Build history of the part. All positions in model axes, mm. A direction names the side the tool comes from. Coordinates: 2 decimals unless noted, no trailing zeros. Loops run counter-clockwise (first coordinate to the right, second up) from the corner with the lowest first, then second, coordinate; pieces in that order, holes last.
(1) Two-plate mould, pull along Y, no slides. Class faces 1 (the face through (41.68, -1.88, -5.96)), 2 (the face through (71.4, -0.1, -13.4)), 3 (the face through (70.4, 6, 5)): pulls with the +Y half, pulls with the -Y half, needs draft (parallel to the pull), parting line crosses it, or undercut.
(2) Slice it at B-B (x = 42). Give the cut face in (y, z), and give its area (3 significant figures).
(3) Slice it at A-A (x = 63). Give the cut face in (y, z), and give its area (3 significant figures).
(4) Wall check: L1, parallel to Y at x = 40.5, z = 3.5; L2, parallel to Z at x = 40, y = -2; L3, parallel to Y at x = 7, z = 0. Give the ranges that are in metal, low to high.
(5) Tool access for faces 4 (the face through (72.16, 6.51, -6.43)), 5 (the face through (35.813, -1.505, 6.777)): list every direction of +Z, -Z, +X, -X, +Y, -Y with a clear straight run to the whole face (end or side of a thin tool).
(6) Flat gauge pins, fed straight in: P1, Ø6, axis at y = 2, z = -0.5, coming from the +X side; P2, Ø6, axis at x = 51, z = 4, coming from the -Y side; P3, Ø4, axis at y = -2.5, z = -2.5, coming from the +X side. Where does each tip first touch, or does it go through?
from build123d import *

# Parameters (mm, degrees)
BOSS_EXTRUDE3_DEPTH = 1.9
FILLET4_R           = 8.6
FILLET5_R           = 0.25
FILLET6_R           = 0.5
FILLET7_R           = 1


with BuildPart() as part:
    # Sketch6 → Boss-Extrude3 (new body)
    with BuildSketch(Plane(origin=(72.3, 0, 0), x_dir=(0, 0, -1), z_dir=(1, 0, 0))):
        with BuildLine():
            Line((-9.834595004, -5.292759782), (0, -9.279892888))
            Line((0, -9.279892888), (9.834595004, -5.292759782))
            ThreePointArc((9.834595004, -5.292759782), (13.4, 0), (9.834595004, 5.292759782))
            Line((9.834595004, 5.292759782), (0, 9.279892888))
            Line((0, 9.279892888), (-9.834595004, 5.292759782))
            ThreePointArc((-9.834595004, 5.292759782), (-13.4, 0), (-9.834595004, -5.292759782))
        make_face()
    extrude(amount=-BOSS_EXTRUDE3_DEPTH)

    # Sketch11 → Revolve1 (revolve)
    with BuildSketch(Plane(origin=(0, 0, 0), x_dir=(-1, 0, 0), z_dir=(0, 0, -1))):
        Polygon((-70.4, 7.131416054), (-70.4, 0), (0, 0), (0, 2), (-8.5, 2.2), (-9.5, 6.85), (-61.4, 7.031165912), (-61.4, 7.1), align=None)
    revolve(axis=Axis((70.4, 0, 0), (-1, 0, 0)))

    # Sketch12 → Hole1 (revolve, cut)
    with BuildSketch(Plane(origin=(72.3, 0, 0), x_dir=(0, 0, -1), z_dir=(0, 1, 0))):
        Polygon((0, 0), (0, 72.3), (1, 72.3), (1, 63.239774349), (6.25, 62.110742091), (6.25, 0), align=None)
    revolve(axis=Axis((78.430023899, 0, 0), (-1, 0, 0)), mode=Mode.SUBTRACT)

    # Fillet4
    fillet4_edges = [part.edges().sort_by_distance(p)[0] for p in [
        (71.35, 9.279892888, 0),
        (71.35, -9.279892888, 0),
    ]]
    fillet(fillet4_edges, radius=FILLET4_R)

    # Fillet5
    fillet5_edges = [part.edges().sort_by_distance(p)[0] for p in [
        (9.060225651, 0, 1),
    ]]
    fillet(fillet5_edges, radius=FILLET5_R)

    # Fillet6
    fillet6_edges = [part.edges().sort_by_distance(p)[0] for p in [
        (70.4, 0, -13.4),
        (70.4, 6.631339679, -6.532876496),
        (70.4, -7.131416054, 0),
        (72.3, -6.631339679, -6.532876496),
        (72.3, 6.631339679, 6.532876496),
        (72.3, 8.6, 0),
        (72.3, -8.6, 0),
        (70.4, -6.631339679, -6.532876496),
        (70.4, 6.631339679, 6.532876496),
        (70.4, 8.6, 0),
        (70.4, -8.6, 0),
        (70.4, 0, 13.4),
        (72.3, 6.631339679, -6.532876496),
        (72.3, 0, -13.4),
        (70.4, -6.631339679, 6.532876496),
        (72.3, -6.631339679, 6.532876496),
        (72.3, 0, 13.4),
    ]]
    fillet(fillet6_edges, radius=FILLET6_R)

    # Fillet7
    fillet7_edges = [part.edges().sort_by_distance(p)[0] for p in [
        (8.5, -2.2, 0),
    ]]
    fillet(fillet7_edges, radius=FILLET7_R)


solid = part.part
Response values:
1. face 1: undercut
1. face 2: parting line crosses it
1. face 3: needs draft
2. outline: circle Ø13.93 at (0, 0); hole circle Ø12.5 at (0, 0)
2. area: 29.6 mm2
3. outline: circle Ø14.21 at (0, 0); hole circle Ø12.5 at (0, 0)
3. area: 35.9 mm2
4. L1: y = -6.01 to -5.18, 5.18 to 6.01
4. L2: z = -6.66 to -5.92, 5.92 to 6.66
4. L3: y = -2.16 to -1, 1 to 2.16
5. face 4: -Z, +X, +Y
5. face 5: -X
6. P1: stops at x = 9.93
6. P2: stops at y = -6.92
6. P3: stops at x = 10.04
